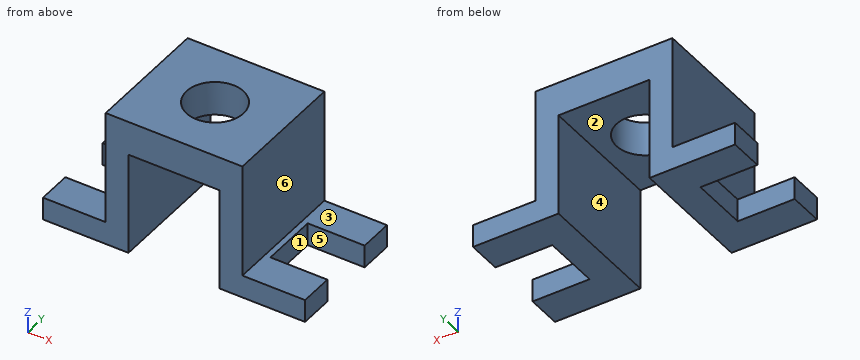
```python
from build123d import *

# Parameters (mm, degrees)
F0_W          = 46
F0_H          = 24
F1_DEPTH      = 11
F1_DEPTH_BACK = 11
F2_W          = 16.6977588087
F2_H          = 22
F2_W_2        = 16
F2_H_2        = 27.9069770836
F3_DEPTH      = 25
F3_DEPTH_BACK = 25
F4_W          = 10
F4_H          = 10
F4_W_2        = 13.8300365831
F4_W_3        = 3.8300365831
F5_DEPTH      = 25
F6_R          = 5
F7_DEPTH      = 10


with BuildPart() as f1:
    # F0 (on Front) → F1 (new body, two sides)
    with BuildSketch(Plane.XZ) as f1_sk:
        Rectangle(F0_W, F0_H)
    extrude(amount=F1_DEPTH)
    extrude(f1_sk.sketch, amount=-F1_DEPTH_BACK)

    # F2 (on Front) → F3 (cut, two sides)
    with BuildSketch(Plane.XZ) as f3_sk:
        with Locations((-20.3488794044, 3)):
            Rectangle(F2_W, F2_H)
        with Locations((20.3488794044, 3)):
            Rectangle(F2_W, F2_H)
        with Locations((0, -7.9534885418)):
            Rectangle(F2_W_2, F2_H_2)
    extrude(amount=-F3_DEPTH, mode=Mode.SUBTRACT)
    extrude(f3_sk.sketch, amount=F3_DEPTH_BACK, mode=Mode.SUBTRACT)

    # F4 (on face) → F5 (cut)
    with BuildSketch(Plane.XY.offset(-8)):
        with Locations((-18, 0)):
            Rectangle(F4_W, F4_H)
        with Locations((19.9150182915, 0)):
            Rectangle(F4_W_2, F4_H)
        with Locations((-24.9150182915, 0)):
            Rectangle(F4_W_3, F4_H)
    extrude(amount=-F5_DEPTH, mode=Mode.SUBTRACT)

    # F6 (on face) → F7 (cut)
    with BuildSketch(Plane.XY.offset(12)):
        Circle(F6_R)
    extrude(amount=-F7_DEPTH, mode=Mode.SUBTRACT)


solid = f1.part
```
Input: part model. Units: mm. Frame: model coordinates. Face numbers are marked on the shaded views. A direction names the side the tool comes from. Give positions to 0.01 mm unless a question says otherwise; leave off trailing zeros. Write each loop counter-clockwise with the first axis right and the second up, starting at its lowest first coordinate (ties: lowest second). Pieces come first, ordered by that corner, then holes. Notation, with made-up numbers: (88, 4) - (93, 4) arc R21 cw to (93, 14) - close; hole circle Ø1 at (-1.5, 71.25). An arc over 180 degrees is marked (long way). Write item = value, one per line. Start each with the question number.
1) Reachability of the marked faces 4, 5 and 6 from +Z, -Z, +X, -X, +Y, -Y: full face, straight path, thin tool, end or side. Return the list, or none.
2) Cut plane C-C (z = 2). Return loops of the section in (x, y), and give its area (3 significant figures).
3) Pin query (flat end, axial travel): pin 1 (1.5 mm diameter, centred on x = 17, y = -5.5, fed in from +Z); pin 2 (4.5 mm diameter, centred on y = 1, z = -9.5, fed in from -X); pin 3 (13 mm diameter, centred on x = 1, y = -5, fed in from -Z). Return the tip coordinate at first contact, or that it passes through.
4) Material intervals for L1, parallel to Y at x = 0, z = 9.35; L2, parallel to X at y = -6.75, z = -5; L3, parallel to X at y = 4, z = -10.5, sorted ascending. Write a range as [from, to].
5) Cut plane A-A (x = -4). Return loops of the section in (y, z).
6) Cut plane B-B (y = 0). Return loops of the section in (x, z).
7) Draft query along X for the marked faces 1, 2 and 3. Return one class per face: pulls with the +X half, pulls with the -X half, needs draft (parallel to the pull), parting line crosses it, or undercut.
8) Cut plane D-D (y = -7). Return loops of the section in (x, z), and give its area (3 significant figures).
Answers follow:
q1.face_4 = -Z, +Y, -Y
q1.face_5 = +Z, -Z, +X
q1.face_6 = +Z, +X, +Y, -Y
q2.outline = (-12, -11) - (-8, -11) - (-8, 11) - (-12, 11) - close; (8, -11) - (12, -11) - (12, 11) - (8, 11) - close
q2.area = 176 mm^2
q3.pin_1 = -8
q3.pin_2 = -13
q3.pin_3 = 6
q4.L1 = [-11, -5], [5, 11]
q4.L2 = [-12, -8], [8, 12]
q4.L3 = [-13, -8], [8, 13]
q5.outline = (-11, 6) - (-3, 6) - (-3, 12) - (-11, 12) - close; (3, 6) - (11, 6) - (11, 12) - (3, 12) - close
q6.outline = (-13, -12) - (-8, -12) - (-8, 6) - (-5, 6) - (-5, 12) - (-12, 12) - (-12, -8) - (-13, -8) - close; (5, 6) - (8, 6) - (8, -12) - (13, -12) - (13, -8) - (12, -8) - (12, 12) - (5, 12) - close
q7.face_1 = pulls with the +X half
q7.face_2 = undercut
q7.face_3 = needs draft
q8.outline = (-23, -12) - (-8, -12) - (-8, 6) - (8, 6) - (8, -12) - (23, -12) - (23, -8) - (12, -8) - (12, 12) - (-12, 12) - (-12, -8) - (-23, -8) - close
q8.area = 376 mm^2
